from build123d import *

# Parameters (mm, degrees)
F1_W     = 69.85
F1_H     = 23.8125
F2_DEPTH = 19.05
F3_T     = -1.5875
F4_R     = 1.5875
F5_DEPTH = 17.4625
F6_R     = 3.175
F7_DEPTH = 1.5875


with BuildPart() as f2:
    # F1 (on Top) → F2 (new body)
    with BuildSketch(Plane.XY):
        with Locations((34.925, 11.90625)):
            Rectangle(F1_W, F1_H)
    extrude(amount=F2_DEPTH)

    # F3
    f3_openings = [f2.faces().sort_by_distance(p)[0] for p in [
        (34.925, 11.90625, 19.05),
    ]]
    offset(amount=F3_T, openings=f3_openings)

    # F4 (on face) → F5 (join, through all)
    with BuildSketch(Plane.XY.offset(19.05)):
        with BuildLine():
            Line((1.5875, 8.5725), (4.191, 8.5725))
            ThreePointArc((4.191, 8.5725), (8.3185, 12.7), (4.191, 16.8275))
            Line((4.191, 16.8275), (1.5875, 16.8275))
            Line((1.5875, 16.8275), (1.5875, 8.5725))
        make_face()
        with Locations((4.191, 12.7)):
            Circle(F4_R, mode=Mode.SUBTRACT)
        with BuildLine():
            Line((65.659, 8.5725), (68.2625, 8.5725))
            Line((68.2625, 8.5725), (68.2625, 16.8275))
            Line((68.2625, 16.8275), (65.659, 16.8275))
            ThreePointArc((65.659, 16.8275), (61.5315, 12.7), (65.659, 8.5725))
        make_face()
        with Locations((65.659, 12.7)):
            Circle(F4_R, mode=Mode.SUBTRACT)
    extrude(amount=-F5_DEPTH)

    # F6 (on face) → F7 (cut, through all)
    with BuildSketch(Plane(origin=(0, 23.8125, 0), x_dir=(-1, 0, 0), z_dir=(0, 1, 0))):
        with Locations((-34.925, 4.7625)):
            Circle(F6_R)
    extrude(amount=-F7_DEPTH, mode=Mode.SUBTRACT)


solid = f2.part
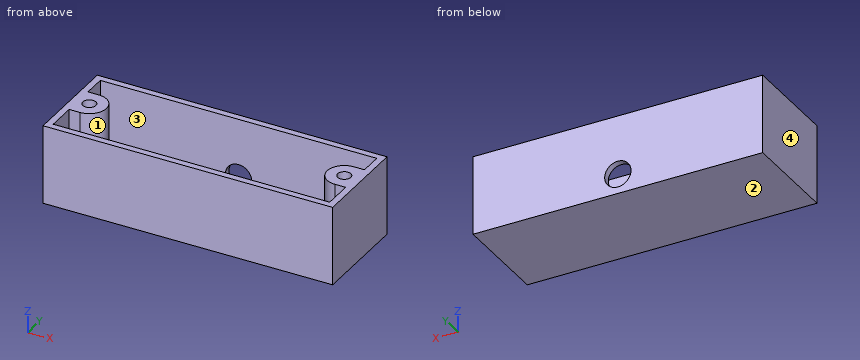
Model file for the job. Use its own axes, mm. Face numbers are marked on the shaded views. Give positions to 0.01 mm unless a question says otherwise; leave off trailing zeros. Order: outer loops, then holes, each group sorted by start corner. A loop starts at its lowest first (then second) coordinate and runs counter-clockwise, first axis right, second up. Notation, with made-up numbers: (14, 73) -> (22, 73) arc R23 ccw to (22, 100) -> close; hole circle Ø9 at (14.5, 43). An arc over 180 degrees is marked (long way). Use CSV: the item, a comma, the result in double quotes.
1. Drill centre lines: line 1 along X through (y, z) = (7.75, 2.25); line 2 along Y through (x, z) = (43, 5.25) (1 decimal); line 3 along Y through (x, z) = (65, 13) (1 decimal). Where is each one in solid material? Low to high. Write a range as from..to.
Outcome:
line 1,"0..1.59, 68.26..69.85"
line 2,"0..1.6, 22.2..23.8"
line 3,"0..1.6, 8.6..11.3, 14.1..16.8, 22.2..23.8"
2. Mould opens along X. For the marked faces 1, 2, 3 and 4 say: +X half, -X half, draft (parallel to the pull), parting line (faces both ways), or undercut.
Outcome:
face 1,"undercut"
face 2,"draft"
face 3,"undercut"
face 4,"-X half"
3. Band-saw the part on D-D, the plane y = 12.7. Give the cut face in (x, z).
Outcome:
outline,"(0, 0) -> (69.85, 0) -> (69.85, 19.05) -> (67.25, 19.05) -> (67.25, 1.59) -> (64.07, 1.59) -> (64.07, 19.05) -> (61.53, 19.05) -> (61.53, 1.59) -> (8.32, 1.59) -> (8.32, 19.05) -> (5.78, 19.05) -> (5.78, 1.59) -> (2.6, 1.59) -> (2.6, 19.05) -> (0, 19.05) -> close"
4. Band-saw the part on A-A, the plane y = 3. Give the cut face in (x, z).
Outcome:
outline,"(0, 0) -> (69.85, 0) -> (69.85, 19.05) -> (68.26, 19.05) -> (68.26, 1.59) -> (1.59, 1.59) -> (1.59, 19.05) -> (0, 19.05) -> close"
5. Drop flat-ended pins along their axis: pin 1 (1 mm diameter, centred on x = 65, y = 12.5, fed in from +Z); pin 2 (4 mm diameter, centred on x = 34.92, z = 4.76, fed in from +Y). Give the stop position or say it passes through.
Outcome:
pin 1,"z = 1.59"
pin 2,"y = 1.59"
6. Band-saw the part on B-B, the plane z = 12. Count the separate pieces of the cut face and the enclosed holes in it, then the cut area to 3 significant figures.
Outcome:
separate pieces,"1"
enclosed holes,"3"
area,"368 mm²"
